Part model, mm, in its own coordinate system. A direction names the side the tool comes from. Coordinates: 2 decimals unless noted, no trailing zeros. Write each loop counter-clockwise with the first axis right and the second up, starting at its lowest first coordinate (ties: lowest second). Pieces come first, ordered by that corner, then holes. Notation, with made-up numbers: (87, 58.5) -> (94, 58.5) arc R17 cw to (94, 86.5) -> close; hole circle Ø11 at (45.5, 70). An arc over 180 degrees is marked (long way). Write item = value, one per line.
from build123d import *

# Parameters (mm, degrees)
SKETCH1_W           = 90
SKETCH1_H           = 64
BOSS_EXTRUDE1_DEPTH = 70
SKETCH2_W           = 26
SKETCH2_H           = 14
CUT_EXTRUDE1_DEPTH  = 90
CUT_EXTRUDE3_START  = -91
CUT_EXTRUDE3_DEPTH  = 92
SKETCH7_R           = 20
CUT_EXTRUDE4_DEPTH  = 48
CUT_EXTRUDE5_START  = -57
CUT_EXTRUDE5_DEPTH  = 66
SKETCH11_W          = 90
SKETCH11_H          = 16
CUT_EXTRUDE7_DEPTH  = 25
SKETCH13_W          = 28
SKETCH13_H          = 16
CUT_EXTRUDE8_DEPTH  = 45


with BuildPart() as part:
    # Sketch1 → Boss-Extrude1 (new body)
    with BuildSketch(Plane(origin=(0, 0, 0), x_dir=(1, 0, 0), z_dir=(0, 1, 0))):
        with Locations((-0.872093023, 32)):
            Rectangle(SKETCH1_W, SKETCH1_H)
    extrude(amount=BOSS_EXTRUDE1_DEPTH)

    # Sketch2 → Cut-Extrude1 (cut)
    with BuildSketch(Plane.ZY.offset(45.872093023)):
        with Locations((-32, 7)):
            Rectangle(SKETCH2_W, SKETCH2_H)
    extrude(amount=-CUT_EXTRUDE1_DEPTH, mode=Mode.SUBTRACT)

    # Sketch3 → Cut-Extrude3 (cut)
    with BuildSketch(Plane.ZY.offset(45.872093023).offset(CUT_EXTRUDE3_START)):
        Polygon((189.287478648, 33), (0, 33), (-8, 33), (-8, 70), (-8, 259.287478648), (277.352473671, 508.070444427), (474.639952319, 281.782965778), align=None)
    cut_extrude3 = extrude(amount=CUT_EXTRUDE3_DEPTH, mode=Mode.SUBTRACT)

    # Mirror2: Cut-Extrude3 across plane
    add(cut_extrude3.mirror(Plane(origin=(0, 0, -32), x_dir=(1, 0, 0), z_dir=(0, 0, -1))), mode=Mode.SUBTRACT)

    # Sketch7 → Cut-Extrude4 (cut)
    with BuildSketch(Plane.XY.offset(-8)):
        with Locations((-0.872093023, 70)):
            Circle(SKETCH7_R)
    extrude(amount=-CUT_EXTRUDE4_DEPTH, mode=Mode.SUBTRACT)

    # Sketch8 → Cut-Extrude5 (cut)
    with BuildSketch(Plane.XY.offset(-8).offset(CUT_EXTRUDE5_START)):
        Polygon((-126.717387311, -166.418392575), (-45.872093023, 33), (-30.872093023, 70), (49.973201264, 269.418392575), (-348.863583887, 431.10898115), (-525.554172461, -4.727804001), align=None)
    cut_extrude5 = extrude(amount=CUT_EXTRUDE5_DEPTH, mode=Mode.SUBTRACT)

    # Mirror3: Cut-Extrude5 across plane
    add(cut_extrude5.mirror(Plane(origin=(-0.872093023, 0, 0), x_dir=(0, 0, 1), z_dir=(1, 0, 0))), mode=Mode.SUBTRACT)

    # Sketch11 → Cut-Extrude7 (cut)
    with BuildSketch(Plane(origin=(0, 70, 0), x_dir=(1, 0, 0), z_dir=(0, 1, 0))):
        with Locations((-0.872093023, 32)):
            Rectangle(SKETCH11_W, SKETCH11_H)
    extrude(amount=-CUT_EXTRUDE7_DEPTH, mode=Mode.SUBTRACT)

    # Sketch13 → Cut-Extrude8 (cut)
    with BuildSketch(Plane(origin=(0, 70, 0), x_dir=(-1, 0, 0), z_dir=(0, -1, 0))):
        with Locations((0.872093023, 8)):
            Rectangle(SKETCH13_W, SKETCH13_H)
    cut_extrude8 = extrude(amount=CUT_EXTRUDE8_DEPTH, mode=Mode.SUBTRACT)

    # Mirror4: Cut-Extrude8 across plane
    add(cut_extrude8.mirror(Plane(origin=(0, 0, -32), x_dir=(1, 0, 0), z_dir=(0, 0, -1))), mode=Mode.SUBTRACT)


solid = part.part
Q1. Saw through at C-C on x = 21. Give the cut face in (y, z), and give its area (3 significant figures).
Model answer:
outline = (0, -64) -> (33, -64) -> (33, -56) -> (70, -56) -> (70, -40) -> (45, -40) -> (45, -24) -> (70, -24) -> (70, -8) -> (33, -8) -> (33, 0) -> (0, 0) -> (0, -19) -> (14, -19) -> (14, -45) -> (0, -45) -> close
area = 3,120 mm²
Q2. Saw through at A-A on y = 60. Give the cut face in (x, z), and give its area (3 significant figures).
Model answer:
outline = (-34.93, -56) -> (-18.19, -56) -> (-18.19, -40) -> (-34.93, -40) -> close; (-34.93, -24) -> (-18.19, -24) -> (-18.19, -8) -> (-34.93, -8) -> close; (16.45, -56) -> (33.18, -56) -> (33.18, -40) -> (16.45, -40) -> close; (16.45, -24) -> (33.18, -24) -> (33.18, -8) -> (16.45, -8) -> close
area = 1,070 mm²
Q3. Probe line 1 (Z direction, x = -7.5, y = 51); line 2 (Y direction, x = 28, z = -4); line 3 (Y direction, x = -12.5, z = -61). List the from-to ranges inside material, lowest first. Write a range as from..to.
Model answer:
line_1 = -48..-40, -24..-16
line_2 = 0..33
line_3 = 0..25
Q4. Saw through at B-B on z = -11. Give the cut face in (x, y), and give its area (3 significant figures).
Model answer:
outline = (-45.87, 0) -> (44.13, 0) -> (44.13, 33) -> (29.13, 70) -> (19.13, 70) arc R20 cw to (13.13, 55.72) -> (13.13, 25) -> (-14.87, 25) -> (-14.87, 55.72) arc R20 cw to (-20.87, 70) -> (-30.87, 70) -> (-45.87, 33) -> close
area = 4,370 mm²
Q5. Saw through at D-D on y = 47. Give the cut face in (x, z).
Model answer:
outline = (-40.2, -56) -> (-14.87, -56) -> (-14.87, -48) -> (13.13, -48) -> (13.13, -56) -> (38.45, -56) -> (38.45, -40) -> (-40.2, -40) -> close; (-40.2, -24) -> (38.45, -24) -> (38.45, -8) -> (13.13, -8) -> (13.13, -16) -> (-14.87, -16) -> (-14.87, -8) -> (-40.2, -8) -> close
Q6. Which spindle directions (+Z, -Z, +X, -X, +Y, -Y) get a long thin tool onto all of the face, cutting with end or side? Do faces 4 (the face through (13.128, 37, -53)), 5 (the face through (-1, 25, -8)), 6 (the face through (-1, 45, -32)), 7 (the face through (-2, 0, -10)), 8 (the face through (-2, 7, -19)). Say none if no direction does.
Model answer:
face_4 = -Z, +Y
face_5 = +Z, +Y
face_6 = +X, -X, +Y
face_7 = +Z, -Z, +X, -X, -Y
face_8 = +X, -X, -Y
Q7. Pin check, flat tips, straight feed: pin 1 (5 mm diameter, centred on x = -29, y = 43, fed in from -Z); pin 2 (5 mm diameter, centred on x = -6.5, z = -6, fed in from +Y); pin 3 (14 mm diameter, centred on x = -4, y = 47, fed in from +Z). Stop position of each tip, or through.
Model answer:
pin_1 = -56
pin_2 = 25
pin_3 = -16
Q8. Mould opens along Z. For faces 1 (the face through (-1, 49, -24)), 2 (the face through (29, 33, -60)), 3 (the face through (25, 48, -56)) say: released by +Z, released by -Z, zero draft, split by the parting line, or undercut.
Model answer:
face_1 = undercut
face_2 = zero draft
face_3 = released by -Z
